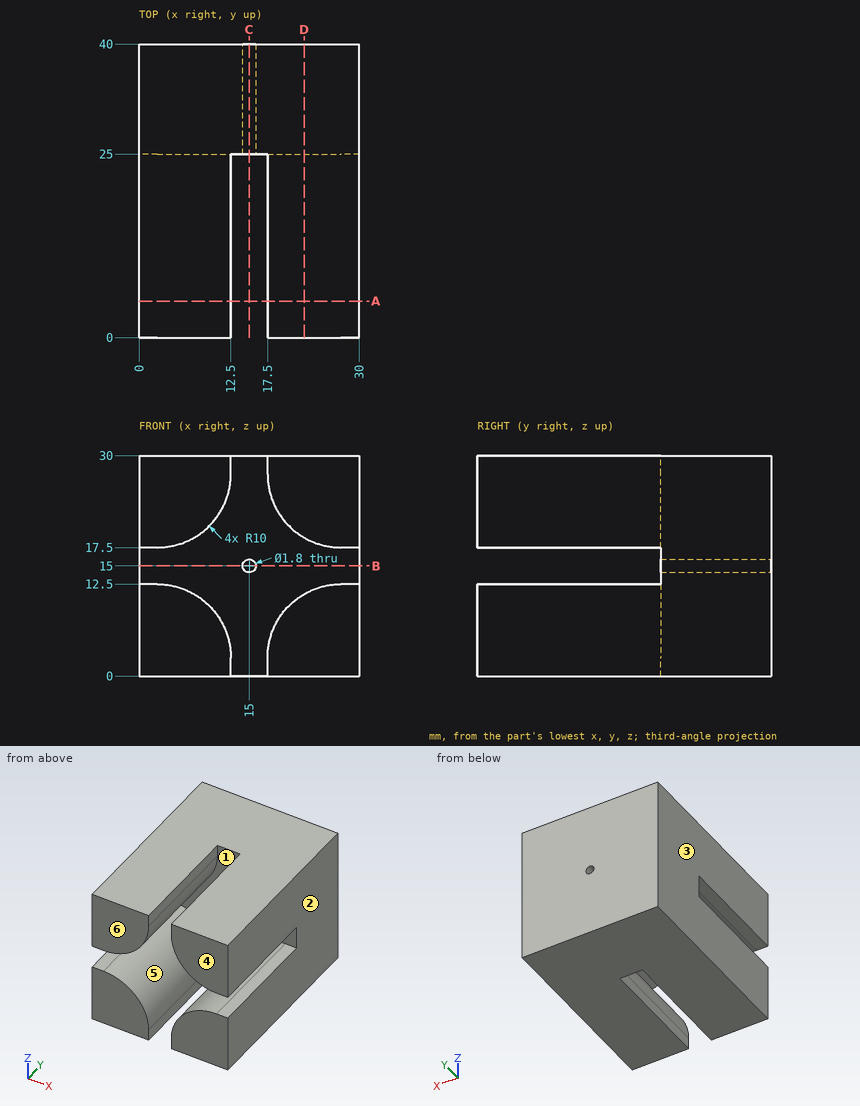
Can you work these out from the drawing? Everything is in mm from the part's minimum corner. A direction names the side the tool comes from. Give positions to 0.01 mm unless a question says otherwise; leave off trailing zeros. Order: outer loops, then holes, each group sorted by start corner. A loop starts at its lowest first (then second) coordinate and runs counter-clockwise, first axis right, second up.
Item 1: For the marked faces 5 and 6, which set-ups out of +Z, -Z, +X, -X, +Y, -Y let a thin tool reach every point of the face, with its end or its side?
Item 2: If we section it at B-B, the plane z = 15: Write out the boundary of the cut face in (x, y), plus the area to 3 significant figures.
Item 3: If we section it at C-C, the plane x = 15: Write out the boundary of the cut face in (y, z), plus the area to 3 significant figures.
Item 4: If we mould it in two halves opening along X, with no side actions, what happens to the marked faces 1, 2, 3 and 4? For each: pulls with the +X half, pulls with the -X half, needs draft (parallel to the pull), parting line crosses it, or undercut.
Item 5: If we section it at D-D, the plane x = 22.5: Write out the boundary of the cut face in (y, z), plus the area to 3 significant figures.
Item 6: If we section it at A-A, the plane y = 5: Write out the boundary of the cut face in (x, z).
Item 7: I'm going to push flat-ended pins straight in: pin 1 (1.5 mm diameter, centred on x = 24, z = 15.5, fed in from -Y); pin 2 (3 mm diameter, centred on x = 15, y = 6, fed in from +Z). Where does each tip first touch, or does it pass through?
Item 8: I need wall thicknesses on line 1 (Z direction, x = 15, y = 28.5); line 2 (Z direction, x = 27.75, y = 15). Which ranges of each line are inside material? Lowest first, please.
Values:
1. face 5: -Y
1. face 6: +Z, -Z, +X, -X, -Y
2. outline: (0, 25) - (14.1, 25) - (14.1, 40) - (0, 40) - close; (15.9, 25) - (30, 25) - (30, 40) - (15.9, 40) - close
2. area: 423 mm2
3. outline: (25, 0) - (40, 0) - (40, 14.1) - (25, 14.1) - close; (25, 15.9) - (40, 15.9) - (40, 30) - (25, 30) - close
3. area: 423 mm2
4. face 1: undercut
4. face 2: pulls with the +X half
4. face 3: pulls with the -X half
4. face 4: needs draft
5. outline: (0, 0) - (40, 0) - (40, 30) - (0, 30) - (0, 18.84) - (25, 18.84) - (25, 11.16) - (0, 11.16) - close
5. area: 1,010 mm2
6. outline: (0, 0) - (12.5, 0) - (12.5, 2.5) arc R10 ccw to (2.5, 12.5) - (0, 12.5) - close; (0, 17.5) - (2.5, 17.5) arc R10 ccw to (12.5, 27.5) - (12.5, 30) - (0, 30) - close; (17.5, 0) - (30, 0) - (30, 12.5) - (27.5, 12.5) arc R10 ccw to (17.5, 2.5) - close; (17.5, 27.5) arc R10 ccw to (27.5, 17.5) - (30, 17.5) - (30, 30) - (17.5, 30) - close
7. pin 1: stops at y = 25
7. pin 2: passes through
8. line 1: z = 0 to 14.1, 15.9 to 30
8. line 2: z = 0 to 12.5, 17.5 to 30
